```python
from build123d import *

# Parameters (mm, degrees)
F2_R = 1.27
F3_R = 1.27


with BuildPart() as f1:
    # F0 (on Front) → F1 (revolve)
    with BuildSketch(Plane.XZ):
        Polygon((-5.8082070693, 3.8550570151), (-6.35, 0), (0, 0), (0, 20.32), (-2.071337691, 20.32), (-2.6532195265, 19.5133350633), (-3.0396357876, 16.7638404987), (-4.5382070693, 15.8119048065), (-3.0396357876, 14.5179457392), (-4.5382070693, 3.8550570151), align=None)
    revolve(axis=Axis((0, 0, 10.16), (0, 0, -1)))

    # F2
    f2_edges = [f1.edges().sort_by_distance(p)[0] for p in [
        (2.071338, 0, 20.32),
        (2.65322, 0, 19.513335),
        (-2.362279, 0, 19.916668),
    ]]
    fillet(f2_edges, radius=F2_R)

    # F3
    f3_edges = [f1.edges().sort_by_distance(p)[0] for p in [
        (5.808207, 0, 3.855057),
        (1.421509, 0, 20.32),
        (4.538207, 0, 15.811905),
        (6.35, 0, 0),
    ]]
    fillet(f3_edges, radius=F3_R)


solid = f1.part
```
Check sheet for the modelled part. Datum: model origin and axes. Units: mm. Round coordinates to 2 decimals unless told otherwise and drop trailing zeros. Order: outer loops, then holes, each group sorted by start corner. A loop starts at its lowest first (then second) coordinate and runs counter-clockwise, first axis right, second up. Notation, with made-up numbers: (81, 26.25) -> (108, 26.25) arc R33 ccw to (108, 54.25) -> close; hole circle Ø4 at (40.25, -31.75). An arc over 180 degrees is marked (long way). One line per item, written item: value. Start each with the question number.
Q1. Thickness scan on line 1 (Z direction, x = 5, y = -1.5); line 2 (Z direction, x = 3, y = 4); line 3 (Y direction, x = -2, z = 17). Record the ranges inside material, lowest first.
Q2. Gauge pin test, flat ends, axial feed: pin 1 Ø6 at (x, z) = (-4.5, 5.5) entering from +Y (3 decimals); pin 2 Ø3 at (x, y) = (-2.5, -2) entering from +Z; pin 3 Ø6 at (x, y) = (0.5, -1) entering from -Z; pin 4 Ø1 at (y, z) = (0.5, 10) entering from +X. Record the tip position at first contact, or that the pin passes through.
Q3. Mould release check, pull along Z, two halves, no side actions. Record for faces 1 (the face through (0, 0, 0)), 2 (the face through (-3.624, 1.141, 9.112)), 3 (the face through (0, 0, 20.32)): pulls with the +Z half, pulls with the -Z half, needs draft (parallel to the pull), parting line crosses it, or undercut.
Q4. Cross-section at A-A (z = 3.5). Record the boundary of the cut face in (x, y) (3 decimals).
Q5. Cross-section at B-B (z = 8.5). Record the boundary of the cut face in (x, y).
Completed:
1. line 1: z = 0.04 to 3.75
1. line 2: z = 0 to 3.82
1. line 3: y = -2.24 to 2.24
2. pin 1: stops at y = 5.215
2. pin 2: stops at z = 20.29
2. pin 3: stops at z = 0
2. pin 4: stops at x = 3.73
3. face 1: pulls with the -Z half
3. face 2: undercut
3. face 3: pulls with the +Z half
4. outline: circle Ø11.17 at (0, 0)
5. outline: circle Ø7.77 at (0, 0)
